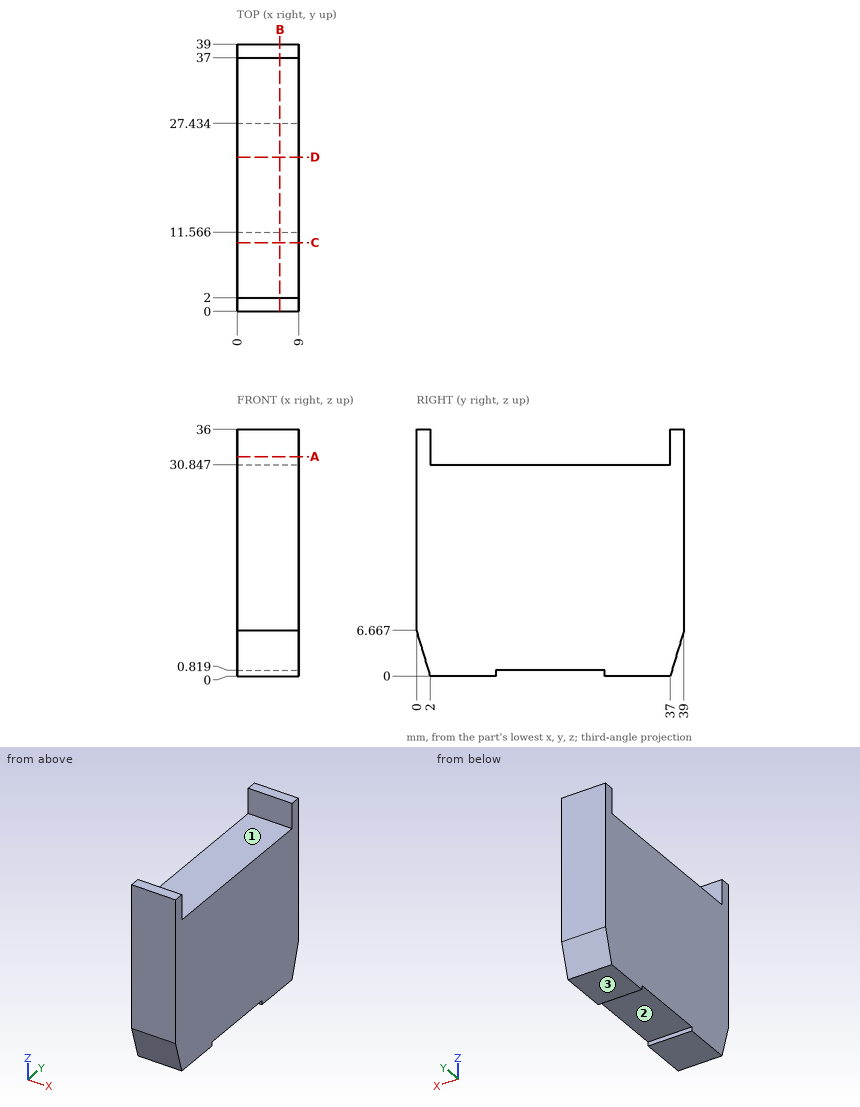
Design review of the part shown in the three views and the two pictorial views. Dimensions are in mm from the part's minimum x, y and z. A direction names the side the tool comes from. Give positions to 0.01 mm unless a question says otherwise; leave off trailing zeros. Loops run counter-clockwise (first coordinate to the right, second up) from the corner with the lowest first, then second, coordinate; pieces in that order, holes last. Notation, with made-up numbers: M 46,-0.75 L 98,-0.75 A6 cw 98,5.25 Z; hole C 21,-36 d9. An arc over 180 degrees is marked long. Put each result on its own line as item: value. Start each with the question number.
(1) Add section B-B, the plane x = 6.25. Write out the cut boundary in (y, z).
(2) Machinability: for the marked faces 1, 2 and 3, which of the approach directions +Z, -Z, +X, -X, +Y, -Y give a long, thin tool a straight path to every point of the face, cutting with its end or side? Answer none if there is none.
(3) Add section C-C, the plane y = 10. Write out the cut boundary in (x, z), then the cut area to 3 significant figures.
(4) Add section D-D, the plane y = 22.5. Write out the cut boundary in (x, z), then the cut area to 3 significant figures.
(5) Add section A-A, the plane z = 32. Write out the cut boundary in (x, y), then the cut area to 3 significant figures.
(6) Wall thickness on L1, parallel to Z at x = 7, y = 34.5; L2, parallel to Z at x = 1.75, y = 20; L3, parallel to Y at x = 1, z = 5: over which ranges is each line inside the solid? List them lowest first.
(7) For pin 1 (4 mm diameter, centred on x = 6, y = 8, fed in from +Z); pin 2 (0.7 mm diameter, centred on x = 5.5, z = 0, fed in from +Y) (1 decimal), all flat-tipped, find the tip position at first contact; note any pin that passes through.
Result:
1. outline: M 0,6.67 L 2,0 L 11.57,0 L 11.57,0.82 L 27.43,0.82 L 27.43,0 L 37,0 L 39,6.67 L 39,36 L 37,36 L 37,30.85 L 2,30.85 L 2,36 L 0,36 Z
2. face 1: +Z, +X, -X
2. face 2: -Z, +X, -X
2. face 3: -Z, +X, -X, +Y, -Y
3. outline: M 0,0 L 9,0 L 9,30.85 L 0,30.85 Z
3. area: 278 mm^2
4. outline: M 0,0.82 L 9,0.82 L 9,30.85 L 0,30.85 Z
4. area: 270 mm^2
5. outline: M 0,0 L 9,0 L 9,2 L 0,2 Z; M 0,37 L 9,37 L 9,39 L 0,39 Z
5. area: 36.0 mm^2
6. L1: z = 0 to 30.85
6. L2: z = 0.82 to 30.85
6. L3: y = 0.5 to 38.5
7. pin 1: stops at z = 30.85
7. pin 2: stops at y = 37.1
